Drawing for the job (mm, zero at the part's lowest x, y, z). A direction names the side the tool comes from. Coordinates: 2 decimals unless noted, no trailing zeros. Write each loop counter-clockwise with the first axis right and the second up, starting at its lowest first coordinate (ties: lowest second). Pieces come first, ordered by that corner, then holes. Notation, with made-up numbers: (-6, 68.5) -> (39, 68.5) arc R22 ccw to (39, 84.5) -> close; hole circle Ø1 at (28, 67). An arc over 180 degrees is marked (long way). Answer as CSV lines item,"result". Start each with the question number.
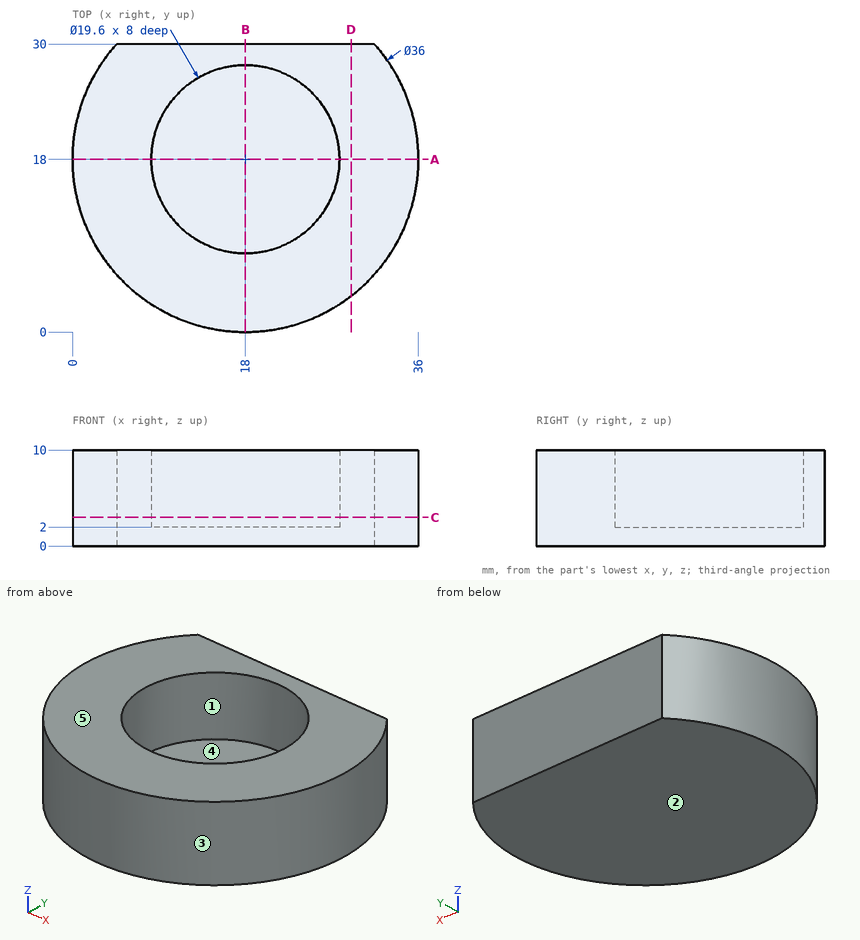
1. Cut at A-A (y = 18). Give the cut face in (x, z), then the cut area to 3 significant figures.
2. Tool access for the marked faces 1 and 2: list every direction of +Z, -Z, +X, -X, +Y, -Y with a clear straight run to the whole face (end or side of a thin tool).
3. Flat gauge pins, fed straight in: P1, Ø5, axis at x = 18, y = 21, coming from the +Z side; P2, Ø5, axis at y = 13, z = 7, coming from the +X side; P3, Ø6, axis at y = 24.5, z = 3.5, coming from the -X side. Where does each tip first touch, or does it go through?
4. Cut at D-D (x = 29). Give the cut face in (y, z), then the cut area to 3 significant figures.
5. Mould opens along X. For the marked faces 3, 4 and 5 say: pulls with the +X half, pulls with the -X half, needs draft (parallel to the pull), parting line crosses it, or undercut.
6. Cut at C-C (z = 3). Give the cut face in (x, y), then the cut area to 3 significant figures.
7. Cut at B-B (x = 18). Give the cut face in (y, z).
8. Wall check: line 1 (X direction, y = 18, z = 6.5); line 2 (Z direction, x = 15, y = 9); line 3 (X direction, y = 22, z = 3). Give the ranges that are in metal, low to high.
Geometry check:
1,outline,"(0, 0) -> (36, 0) -> (36, 10) -> (27.8, 10) -> (27.8, 2) -> (8.2, 2) -> (8.2, 10) -> (0, 10) -> close"
1,area,"203 mm²"
2,face 1,"+Z"
2,face 2,"-Z, +X, -X, +Y, -Y"
3,P1,"z = 2"
3,P2,"x = 35.83"
3,P3,"x = 0.34"
4,outline,"(3.75, 0) -> (30, 0) -> (30, 10) -> (3.75, 10) -> close"
4,area,"262 mm²"
5,face 3,"parting line crosses it"
5,face 4,"undercut"
5,face 5,"needs draft"
6,outline,"(4.58, 30) arc R18 ccw (long way) to (31.42, 30) -> close; hole circle Ø19.6 at (18, 18)"
6,area,"605 mm²"
7,outline,"(0, 0) -> (30, 0) -> (30, 10) -> (27.8, 10) -> (27.8, 2) -> (8.2, 2) -> (8.2, 10) -> (0, 10) -> close"
8,line 1,"0 to 8.2, 27.8 to 36"
8,line 2,"0 to 2"
8,line 3,"0.45 to 9.05, 26.95 to 35.55"
